from build123d import *

# Parameters (mm, degrees)
SKETCH1_R               = 2.5273
BOSS_EXTRUDE1_DEPTH     = 2.794
F_2_CLEARANCE_HOLE1_D   = 2.4384
FILLET1_R               = 2.54
CUT_EXTRUDE2_DEPTH      = 58.306278691
CUT_EXTRUDE2_DEPTH_BACK = 58.306278691


with BuildPart() as part:
    # Sketch1 → Boss-Extrude1 (new, symmetric)
    with BuildSketch(Plane.XY):
        with BuildLine():
            Line((-23.865093494, -0.254), (-47.625, -12.7))
            Line((-47.625, -12.7), (-47.625, -31.75))
            Line((-47.625, -31.75), (47.625, -31.75))
            Line((47.625, -31.75), (47.625, -12.7))
            Line((47.625, -12.7), (23.865093494, -0.254))
            Line((23.865093494, -0.254), (23.865093494, 0))
            ThreePointArc((23.865093494, 0), (0, 23.865093494), (-23.865093494, 0))
            Line((-23.865093494, 0), (-23.865093494, -0.254))
        make_face()
        Circle(SKETCH1_R, mode=Mode.SUBTRACT)
    extrude(amount=BOSS_EXTRUDE1_DEPTH, both=True)

    # #2 Clearance Hole1 (through all)
    with Locations(Plane.XY.offset(2.794)):
        with Locations((-15.875, 0)):
            Hole(F_2_CLEARANCE_HOLE1_D / 2)

    # Fillet1
    fillet1_edges = [part.edges().sort_by_distance(p)[0] for p in [
        (47.625, -12.7, 0),
        (23.865093494, -0.254, 0),
        (-47.625, -12.7, 0),
        (-23.865093494, -0.254, 0),
    ]]
    fillet(fillet1_edges, radius=FILLET1_R)

    # Sketch6 → Cut-Extrude2 (cut, two sides: drawn at the far end of the back side and taken through both)
    with BuildSketch(Plane.XY.offset(-CUT_EXTRUDE2_DEPTH_BACK)):
        Polygon((-27.78125, -31.75), (-27.78125, -26.19375), (-30.1625, -26.19375), (-30.1625, -21.43125), (-27.78125, -21.43125), (-27.78125, -15.875), (-23.01875, -15.875), (-23.01875, -21.43125), (-20.6375, -21.43125), (-20.6375, -26.19375), (-23.01875, -26.19375), (-23.01875, -31.75), align=None)
        Polygon((23.01875, -31.75), (23.01875, -26.19375), (20.6375, -26.19375), (20.6375, -21.43125), (23.01875, -21.43125), (23.01875, -15.875), (27.78125, -15.875), (27.78125, -21.43125), (30.1625, -21.43125), (30.1625, -26.19375), (27.78125, -26.19375), (27.78125, -31.75), align=None)
    extrude(amount=CUT_EXTRUDE2_DEPTH + CUT_EXTRUDE2_DEPTH_BACK, mode=Mode.SUBTRACT)


solid = part.part
For this review, take the finished solid that the model builds, in its own axes (mm). A direction names the side the tool comes from. Give positions to 0.01 mm unless a question says otherwise; leave off trailing zeros. Loops run counter-clockwise (first coordinate to the right, second up) from the corner with the lowest first, then second, coordinate; pieces in that order, holes last.
Item 1: Draft analysis for pull direction X (two halves, no side actions). For faces 4 (the flat face through (-22, -21.431, 0)), 5 (the flat face through (-1, -10, -2.794)), 6 (the flat face through (-47.625, -23, 0)), 7 (the flat face through (-27.781, -19, 0)), state which applies: +X half, -X half, draft (parallel to the pull), parting line (faces both ways), or undercut.
Item 2: Take a section at B-B, the plane x = 0. State the section outline as (y, z) points, and give its area (3 significant figures).
Item 3: Take a section at D-D, the plane x = -36.5. State the section outline as (y, z) points, and give its area (3 significant figures).
Item 4: Insertion check: pin 1 (1.2 mm diameter, centred on x = 22.5, z = 1, fed in from +Y); pin 2 (1 mm diameter, centred on y = 16, z = 2, fed in from +X); pin 3 (0.7 mm diameter, centred on x = 29, z = -1, fed in from +Y). Each pin has a flat end and moves straight along its axis. Give the tip position at first contact, or say it passes through.
Item 5: Tool access review of faces 1 (the cylindrical face through (47.27, -12.94, 0.04)), 2 (the flat face through (-27.781, -29, 0)), 3 (the flat face through (-22, -26.194, 0)): name each direction out of +Z, -Z, +X, -X, +Y, -Y from which nothing blocks a thin tool from reaching the whole face with its end or side.
Item 6: Take a section at A-A, the plane y = -28. State the section outline as (x, z) points (3 decimals).
Item 7: For line 1 along X through (y, z) = (-26, -0.25) (1 decimal); line 2 along Y through (x, z) = (0, 0.05); line 3 along X through (y, z) = (-26.5, -1.6) (3 decimals), list the stretches that pass through material, from the lowest coordinate up.
Item 8: Take a section at C-C, the plane z = 0.45. Give the number of separate pieces and of enclosed holes in the cut face, and give its area (3 significant figures).
Calculated:
1. face 4: undercut
1. face 5: draft
1. face 6: -X half
1. face 7: undercut
2. outline: (-31.75, -2.79) - (-2.53, -2.79) - (-2.53, 2.79) - (-31.75, 2.79) - close; (2.53, -2.79) - (23.87, -2.79) - (23.87, 2.79) - (2.53, 2.79) - close
2. area: 283 mm2
3. outline: (-31.75, -2.79) - (-6.87, -2.79) - (-6.87, 2.79) - (-31.75, 2.79) - close
3. area: 139 mm2
4. pin 1: stops at y = 9.48
4. pin 2: stops at x = 18.15
4. pin 3: stops at y = -2.76
5. face 1: +Z, -Z, +X, +Y
5. face 2: +Z, -Z, -Y
5. face 3: +Z, -Z
6. outline: (-47.625, -2.794) - (-27.781, -2.794) - (-27.781, 2.794) - (-47.625, 2.794) - close; (-23.019, -2.794) - (23.019, -2.794) - (23.019, 2.794) - (-23.019, 2.794) - close; (27.781, -2.794) - (47.625, -2.794) - (47.625, 2.794) - (27.781, 2.794) - close
7. line 1: x = -47.6 to -30.2, -20.6 to 20.6, 30.2 to 47.6
7. line 2: y = -31.75 to -2.53, 2.53 to 23.87
7. line 3: x = -47.625 to -27.781, -23.019 to 23.019, 27.781 to 47.625
8. separate pieces: 1
8. enclosed holes: 2
8. area: 3,390 mm2
